Check sheet for the modelled part. Datum: model origin and axes. Units: mm. A direction names the side the tool comes from. Give positions to 0.01 mm unless a question says otherwise; leave off trailing zeros. Order: outer loops, then holes, each group sorted by start corner. A loop starts at its lowest first (then second) coordinate and runs counter-clockwise, first axis right, second up.
```python
from build123d import *

# Parameters (mm, degrees)
BOSS_EXTRUDE1_DEPTH = 3
CUT_EXTRUDE1_DEPTH  = 3
SKETCH4_W           = 16
SKETCH4_H           = 5
BOSS_EXTRUDE2_DEPTH = 45
BOSS_EXTRUDE3_DEPTH = 16
SKETCH8_W           = 0.849028348
SKETCH8_H           = 44.071161876
SKETCH8_W_2         = 1.029765792
BOSS_EXTRUDE4_DEPTH = 1
BOSS_EXTRUDE5_DEPTH = 3


with BuildPart() as part:
    # Sketch1 → Boss-Extrude1 (new body)
    with BuildSketch(Plane.XY):
        Polygon((0, 0), (120, 0), (120, 10), (75, 10), (68, 17), (68, 40), (68, 90), (52, 90), (52, 40), (52, 17), (45, 10), (0, 10), align=None)
    extrude(amount=BOSS_EXTRUDE1_DEPTH)

    # Sketch2 → Cut-Extrude1 (cut)
    with BuildSketch(Plane.XY.offset(3)):
        with BuildLine():
            Line((3.5, 7.1), (10.5, 7.1))
            ThreePointArc((10.5, 7.1), (12.6, 5), (10.5, 2.9))
            Line((10.5, 2.9), (3.5, 2.9))
            ThreePointArc((3.5, 2.9), (1.4, 5), (3.5, 7.1))
        make_face()
        with BuildLine():
            Line((31.5, 7.1), (38.5, 7.1))
            ThreePointArc((38.5, 7.1), (40.6, 5), (38.5, 2.9))
            Line((38.5, 2.9), (31.5, 2.9))
            ThreePointArc((31.5, 2.9), (29.4, 5), (31.5, 7.1))
        make_face()
        with BuildLine():
            Line((81.5, 7.1), (88.5, 7.1))
            ThreePointArc((88.5, 7.1), (90.6, 5), (88.5, 2.9))
            Line((88.5, 2.9), (81.5, 2.9))
            ThreePointArc((81.5, 2.9), (79.4, 5), (81.5, 7.1))
        make_face()
        with BuildLine():
            Line((116.5, 2.9), (109.5, 2.9))
            ThreePointArc((109.5, 2.9), (107.4, 5), (109.5, 7.1))
            Line((109.5, 7.1), (116.5, 7.1))
            ThreePointArc((116.5, 7.1), (118.6, 5), (116.5, 2.9))
        make_face()
    extrude(amount=-CUT_EXTRUDE1_DEPTH, mode=Mode.SUBTRACT)

    # Sketch4 → Boss-Extrude2 (add)
    with BuildSketch(Plane(origin=(0, 0, 0), x_dir=(-1, 0, 0), z_dir=(0, 0, -1))):
        with Locations((-60, 87.5)):
            Rectangle(SKETCH4_W, SKETCH4_H)
    extrude(amount=BOSS_EXTRUDE2_DEPTH)

    # Sketch7 → Boss-Extrude3 (add)
    with BuildSketch(Plane.ZY.offset(-52)):
        Polygon((-22.5, 85), (0, 62.5), (0, 65.90318292), (-19.09681708, 85), align=None)
    extrude(amount=-BOSS_EXTRUDE3_DEPTH)

    # Sketch8 → Boss-Extrude4 (add)
    with BuildSketch(Plane(origin=(0, 0, 0), x_dir=(-1, 0, 0), z_dir=(0, 0, -1))):
        with Locations((-56.917783528, 39.035580938)):
            Rectangle(SKETCH8_W, SKETCH8_H)
        with Locations((-63.407411106, 39.035580938)):
            Rectangle(SKETCH8_W_2, SKETCH8_H)
    extrude(amount=BOSS_EXTRUDE4_DEPTH)

    # Sketch9 → Boss-Extrude5 (add)
    with BuildSketch(Plane.XY.offset(3)):
        Polygon((22.5, 10), (52, 53.5), (52, 56.880398444), (20.207545882, 10), align=None)
        Polygon((97.5, 10), (68, 53.5), (68, 56.880398444), (99.792454118, 10), align=None)
    extrude(amount=-BOSS_EXTRUDE5_DEPTH)


solid = part.part
```
(1) Gauge pin test, flat ends, axial feed: pin 1 Ø4 at (x, z) = (25.5, -3) entering from +Y; pin 2 Ø0.9 at (x, z) = (14.5, 2) entering from +Y; pin 3 Ø0.7 at (x, y) = (57, 33) entering from -Z; pin 4 Ø0.8 at (y, z) = (33, -0.5) entering from +X. Record the tip position at first contact, or that the pin passes through.
Response values:
pin 1: passes through
pin 2: stops at y = 10
pin 3: stops at z = -1
pin 4: stops at x = 63.92
(2) Cross-section at C-C on y = 13.5. Enter the section's corners in (x, z), then the cut area to 3 significant figures.
Response values:
outline: (22.58, 0) - (24.87, 0) - (24.87, 3) - (22.58, 3) - close; (48.5, 0) - (71.5, 0) - (71.5, 3) - (48.5, 3) - close; (95.13, 0) - (97.42, 0) - (97.42, 3) - (95.13, 3) - close
area: 82.8 mm2
(3) Release check for a two-part mould opening along X. For faces 5 (the face through (35, 7.1, 2)), 6 (the face through (0, 5, 1)), 7 (the face through (59.9, 73.9, -11.4)), 8 (the face through (83.674, 33.768, 1.521)) record: released by +X, released by -X, zero draft, split by the parting line, or undercut.
Response values:
face 5: undercut
face 6: released by -X
face 7: zero draft
face 8: released by +X
(4) Set-up check for faces 1 (the face through (60, 88, -45)), 2 (the face through (110, 10, 1)), 3 (the face through (60, 85, -9)), 4 (the face through (107.4, 5, 1.5)): record each of +Z, -Z, +X, -X, +Y, -Y from which the full face is reachable in a straight line by a thin tool's end or side.
Response values:
face 1: -Z, +X, -X, +Y, -Y
face 2: +Z, -Z, +X, +Y
face 3: +X, -X
face 4: +Z, -Z
(5) Cross-section at D-D on y = 46. Enter the section's corners in (x, z).
Response values:
outline: (44.62, 0) - (46.91, 0) - (46.91, 3) - (44.62, 3) - close; (52, 0) - (56.49, 0) - (56.49, -1) - (57.34, -1) - (57.34, 0) - (62.89, 0) - (62.89, -1) - (63.92, -1) - (63.92, 0) - (68, 0) - (68, 3) - (52, 3) - close; (73.09, 0) - (75.38, 0) - (75.38, 3) - (73.09, 3) - close
(6) Material ranges on L1, parallel to X at y = 86.5, z = -8; L2, parallel to Z at x = 54, y = 51.5; L3, parallel to Z at x = 67, y = 69, recorded low to high.
Response values:
L1: x = 52 to 68
L2: z = 0 to 3
L3: z = -6.5 to -3.1, 0 to 3
(7) Cross-section at A-A on x = 9. Enter the section's corners in (y, z).
Response values:
outline: (0, 0) - (2.9, 0) - (2.9, 3) - (0, 3) - close; (7.1, 0) - (10, 0) - (10, 3) - (7.1, 3) - close
(8) Cross-section at B-B on z = -15.5. Enter the section's corners in (x, y).
Response values:
outline: (52, 78) - (68, 78) - (68, 81.4) - (52, 81.4) - close; (52, 85) - (68, 85) - (68, 90) - (52, 90) - close
